Model file for the job. Use its own axes, mm. Round coordinates to 2 decimals unless told otherwise and drop trailing zeros. Loops run counter-clockwise (first coordinate to the right, second up) from the corner with the lowest first, then second, coordinate; pieces in that order, holes last. Notation, with made-up numbers: M 62,20 L 91,20 A24 cw 91,51 Z; hole C 13,82 d8. An arc over 180 degrees is marked long. Use a Markdown table: item, result. Add a question column.
Q1. Mould opens along Y. For faces 1 (the face through (5, -2.206, 74)), 2 (the face through (4.97, -7.38, 73.95)), 3 (the face through (0, -3.589, 74)) say: +Y half, -Y half, draft (parallel to the pull), parting line (faces both ways), or undercut.
Q2. Pin check, flat tips, straight feed: pin 1 (4 mm diameter, centred on x = -1, z = 65.5, fed in from +Y); pin 2 (1 mm diameter, centred on y = -6, z = 35.5, fed in from -X). Stop position of each tip, or through.
Q3. Cut at B-B (z = 56.5). Give the cut face in (x, y), plus the area to 3 significant figures.
Q4. Probe line 1 (Y direction, x = 0, z = 112); line 2 (X direction, y = -2.75, z = 84.5); line 3 (Y direction, x = -2.75, z = 60). List the from-to ranges inside material, lowest first. Write a range as from..to.
Q5. Cut at C-C (x = -5.75). Give the cut face in (y, z), plus the area to 3 significant figures.
Q6. Cut at A-A (y = -6.5). Give the cut face in (x, z), plus the area to 3 significant figures.
from build123d import *

# Parameters (mm, degrees)
F1_DEPTH = 150


with BuildPart() as f1:
    # F0 (on Top) → F1 (new body)
    with BuildSketch(Plane.XY):
        Polygon((7, -5.088528), (7, -3.588528), (4.5, -3.588528), (-4.5, -3.588528), (-7, -3.588528), (-7, -5.088528), align=None)
        Polygon((4.5, -3.588528), (7, -3.588528), (7, -2.205549), (3.339543, -2.205549), align=None)
        with BuildLine():
            Line((3, -9.604092), (7, -5.088528))
            Line((7, -5.088528), (-7, -5.088528))
            Line((-7, -5.088528), (-3, -9.604092))
            Line((-3, -9.604092), (-1, -9.604092))
            ThreePointArc((-1, -9.604092), (0, -5.338528), (1, -9.604092))
            Line((1, -9.604092), (3, -9.604092))
        make_face()
        Polygon((-7, -3.588528), (-4.5, -3.588528), (-3.339543, -2.205549), (-7, -2.205549), align=None)
    extrude(amount=F1_DEPTH)


solid = f1.part
Checked values:
| question | item | result |
|---|---|---|
| 1 | face 1 | +Y half |
| 1 | face 2 | -Y half |
| 1 | face 3 | undercut |
| 2 | pin 1 | stops at y = -3.59 |
| 2 | pin 2 | stops at x = -6.64 |
| 3 | outline | M -7,-5.09 L -3,-9.6 L -1,-9.6 A2.25 cw long 1,-9.6 L 3,-9.6 L 7,-5.09 L 7,-2.21 L 3.34,-2.21 L 4.5,-3.59 L -4.5,-3.59 L -3.34,-2.21 L -7,-2.21 Z |
| 3 | area | 59.1 mm^2 |
| 4 | line 1 | y = -5.34..-3.59 |
| 4 | line 2 | x = -7..-3.8, 3.8..7 |
| 4 | line 3 | y = -9.6..-3.59 |
| 5 | outline | M -6.5,0 L -2.21,0 L -2.21,150 L -6.5,150 Z |
| 5 | area | 644 mm^2 |
| 6 | outline | M -5.75,0 L -1.97,0 L -1.97,150 L -5.75,150 Z; M 1.97,0 L 5.75,0 L 5.75,150 L 1.97,150 Z |
| 6 | area | 1,130 mm^2 |
